Autodesk Inventor part; units mm, degrees
ref_plane "YZ Plane" through (0, 0, 0) normal (1, 0, 0) x (0, 1, 0)
ref_plane "XZ Plane" through (0, 0, 0) normal (0, 1, 0) x (-1, 0, 0)
ref_plane "XY Plane" through (0, 0, 0) normal (0, 0, 1) x (1, 0, 0)
sketch "Sketch1" plane through (0, 0, 0) normal (0, 0, 1) x (1, 0, 0)
  line L0 (0, 0) -> (76.2, 0)
  line L1 (76.2, 0) -> (76.2, 25.4)
  line L2 (76.2, 25.4) -> (50.8, 101.6)
  line L3 (50.8, 101.6) -> (25.4, 101.6)
  line L4 (25.4, 101.6) -> (0, 25.4)
  line L5 (0, 25.4) -> (0, 0)
  line L6 (0, 25.4) -> (76.2, 25.4) construction
  line L7 (25.4, 101.6) -> (25.4, 25.4) construction
  line L8 (50.8, 101.6) -> (50.8, 25.4) construction
  circle A0 centre (12.7, 12.7) radius 1.5875
  circle A1 centre (25.4, 12.7) radius 1.5875
  circle A2 centre (38.1, 12.7) radius 1.5875
  circle A3 centre (50.8, 12.7) radius 1.5875
  circle A4 centre (63.5, 12.7) radius 1.5875
  circle A5 centre (38.1, 88.7759) radius 1.5875
  circle A6 centre (38.1, 76.0759) radius 1.5875
  circle A7 centre (38.1, 63.3759) radius 1.5875
  circle A8 centre (38.1, 50.6759) radius 1.5875
  circle A9 centre (38.1, 37.9759) radius 1.5875
  dimension "d0" = 25.4
  dimension "d1" = 76.2
  dimension "d2" = 101.6
  dimension "d3" = 12.7
  dimension "d4" = 12.7
  dimension "d7" = 12.7
  dimension "d12" = 3.175
  dimension "d13" = 12.8241
  dimension "d14" = 12.7
  dimension "d17" = 12.7
extrude "Extrusion1" add sketch "Sketch1" along normal blind 3.175
equation "\"d4\" = d3"
properties part number "8 ball frame gusset"
The model under review builds one solid part; all positions refer to its coordinate system, in mm. Give positions to 0.01 mm unless a question says otherwise; leave off trailing zeros. Write each loop counter-clockwise with the first axis right and the second up, starting at its lowest first coordinate (ties: lowest second). Pieces come first, ordered by that corner, then holes.
1. Add section C-C, the plane x = 38.1. Write out the cut boundary in (y, z) (1 decimal), plus the area to 3 significant figures.
2. Draft analysis for pull direction X (two halves, no side actions). For faces 1 (the flat face through (76.2, 13, 2)), 2 (the flat face through (0, 13, 2)), 3 (the cylindrical face through (37.756, 52.226, 1.565)), state which applies: +X half, -X half, draft (parallel to the pull), parting line (faces both ways), or undercut.
3. Add section D-D, the plane z = 2.35. Count the separate pieces of the cut face and the enclosed holes in it, plus the area to 3 significant figures.
4. Add section B-B, the plane y = 12.7. Write out the cut boundary in (x, z) (1 decimal), plus the area to 3 significant figures.
5. Wall thickness on L1, parallel to X at y = 52, z = 1; L2, parallel to X at y = 32.5, z = 1.05; L3, parallel to X at y = 97, z = 2.55: over which ranges is each line inside the solid? List them lowest first.
6. Add section A-A, the plane x = 12.7. Write out the cut boundary in (y, z) (1 decimal).
7. For P1, Ø5, axis at x = 25.4, y = 12.7, coming from the -Z side; P2, Ø1, axis at y = 27.5, z = 2, coming from the +X side, all flat-tipped, find the tip position at first contact; note any pin that passes through.
Worked answers:
1. outline: (0, 0) - (11.1, 0) - (11.1, 3.2) - (0, 3.2) - close; (14.3, 0) - (36.4, 0) - (36.4, 3.2) - (14.3, 3.2) - close; (39.6, 0) - (49.1, 0) - (49.1, 3.2) - (39.6, 3.2) - close; (52.3, 0) - (61.8, 0) - (61.8, 3.2) - (52.3, 3.2) - close; (65, 0) - (74.5, 0) - (74.5, 3.2) - (65, 3.2) - close; (77.7, 0) - (87.2, 0) - (87.2, 3.2) - (77.7, 3.2) - close; (90.4, 0) - (101.6, 0) - (101.6, 3.2) - (90.4, 3.2) - close
1. area: 262 mm2
2. face 1: +X half
2. face 2: -X half
2. face 3: undercut
3. separate pieces: 1
3. enclosed holes: 10
3. area: 5,730 mm2
4. outline: (0, 0) - (11.1, 0) - (11.1, 3.2) - (0, 3.2) - close; (14.3, 0) - (23.8, 0) - (23.8, 3.2) - (14.3, 3.2) - close; (27, 0) - (36.5, 0) - (36.5, 3.2) - (27, 3.2) - close; (39.7, 0) - (49.2, 0) - (49.2, 3.2) - (39.7, 3.2) - close; (52.4, 0) - (61.9, 0) - (61.9, 3.2) - (52.4, 3.2) - close; (65.1, 0) - (76.2, 0) - (76.2, 3.2) - (65.1, 3.2) - close
4. area: 192 mm2
5. L1: x = 8.87 to 37.22, 38.98 to 67.33
5. L2: x = 2.37 to 73.83
5. L3: x = 23.87 to 52.33
6. outline: (0, 0) - (11.1, 0) - (11.1, 3.2) - (0, 3.2) - close; (14.3, 0) - (63.5, 0) - (63.5, 3.2) - (14.3, 3.2) - close
7. P1: stops at z = 0
7. P2: stops at x = 75.67
